```python
from build123d import *

# Parameters (mm, degrees)
SKETCH2_R               = 11.43
BOSS_EXTRUDE1_DEPTH     = 6.35
SKETCH4_R               = 1.5
CUT_EXTRUDE1_DEPTH      = 18.366988801
CUT_EXTRUDE2_REACH      = 29.445
CUT_EXTRUDE2_END_RADIUS = 1.5
CUT_EXTRUDE3_REACH      = 29.445
CUT_EXTRUDE3_END_RADIUS = 1.5
SKETCH9_R               = 1
SKETCH10_R              = 5.08
CUT_EXTRUDE4_DEPTH      = 3.81


with BuildPart() as part:
    # Sketch2 → Boss-Extrude1 (new body)
    with BuildSketch(Plane(origin=(0, 0, 0), x_dir=(1, 0, 0), z_dir=(0, 1, 0))):
        with Locations(Location((0, 0, 0), (0, 0, 270))):
            Circle(SKETCH2_R)
    extrude(amount=BOSS_EXTRUDE1_DEPTH)

    # Sketch4 → Cut-Extrude1 (cut, through all)
    with BuildSketch(Plane(origin=(0, 6.35, 0), x_dir=(1, 0, 0), z_dir=(0, 1, 0))):
        with Locations(Location((0, 8, 0), (0, 0, 270))):
            Circle(SKETCH4_R)
        with Locations(Location((0, -8, 0), (0, 0, 270))):
            Circle(SKETCH4_R)
        with Locations(Location((9.5, 0, 0), (0, 0, 270))):
            Circle(SKETCH4_R)
        with Locations(Location((-9.5, 0, 0), (0, 0, 270))):
            Circle(SKETCH4_R)
    extrude(amount=-CUT_EXTRUDE1_DEPTH, mode=Mode.SUBTRACT)

    # Cut-Extrude2: up to this cylinder (the profile starts outside it)
    cut_extrude2_end = Plane(origin=(0, 3.175, 8), z_dir=(0, 1, 0)) * Cylinder(CUT_EXTRUDE2_END_RADIUS, 62.89, mode=Mode.PRIVATE)
    # Sketch8 → Cut-Extrude2 (cut, up to the surface)
    with BuildSketch(Plane.XY.offset(12.7), mode=Mode.PRIVATE) as cut_extrude2_sk1:
        with BuildLine():
            ThreePointArc((1, 3.175), (0.707106781, 3.882106781), (0, 4.175))
            Line((0, 4.175), (0, 2.175))
            ThreePointArc((0, 2.175), (0.707106781, 2.467893219), (1, 3.175))
        make_face()
    cut_extrude2_tool1 = extrude(cut_extrude2_sk1.sketch, amount=-CUT_EXTRUDE2_REACH, mode=Mode.PRIVATE) - cut_extrude2_end
    add(cut_extrude2_tool1.solids().sort_by_distance((0.424413, 3.175, 12.7))[0], mode=Mode.SUBTRACT)
    # Sketch8 → Cut-Extrude2 (cut, up to the surface)
    with BuildSketch(Plane.XY.offset(12.7), mode=Mode.PRIVATE) as cut_extrude2_sk2:
        with BuildLine():
            Line((0, 2.175), (0, 4.175))
            ThreePointArc((0, 4.175), (-1, 3.175), (0, 2.175))
        make_face()
    cut_extrude2_tool2 = extrude(cut_extrude2_sk2.sketch, amount=-CUT_EXTRUDE2_REACH, mode=Mode.PRIVATE) - cut_extrude2_end
    add(cut_extrude2_tool2.solids().sort_by_distance((-0.424413, 3.175, 12.7))[0], mode=Mode.SUBTRACT)
    # Sketch8 → Cut-Extrude2 (cut, up to the surface)
    with BuildSketch(Plane.XY.offset(12.7), mode=Mode.PRIVATE) as cut_extrude2_sk3:
        with BuildLine():
            ThreePointArc((1, 3.175), (0.707106781, 3.882106781), (0, 4.175))
            Line((0, 4.175), (0, 2.175))
            ThreePointArc((0, 2.175), (0.707106781, 2.467893219), (1, 3.175))
        make_face()
    cut_extrude2_tool3 = extrude(cut_extrude2_sk3.sketch, amount=-CUT_EXTRUDE2_REACH, mode=Mode.PRIVATE) - cut_extrude2_end
    add(cut_extrude2_tool3.solids().sort_by_distance((0.424413, 3.175, 12.7))[0], mode=Mode.SUBTRACT)
    # Sketch8 → Cut-Extrude2 (cut, up to the surface)
    with BuildSketch(Plane.XY.offset(12.7), mode=Mode.PRIVATE) as cut_extrude2_sk4:
        with BuildLine():
            Line((0, 2.175), (0, 4.175))
            ThreePointArc((0, 4.175), (-1, 3.175), (0, 2.175))
        make_face()
    cut_extrude2_tool4 = extrude(cut_extrude2_sk4.sketch, amount=-CUT_EXTRUDE2_REACH, mode=Mode.PRIVATE) - cut_extrude2_end
    add(cut_extrude2_tool4.solids().sort_by_distance((-0.424413, 3.175, 12.7))[0], mode=Mode.SUBTRACT)

    # Cut-Extrude3: up to this cylinder (the profile starts outside it)
    cut_extrude3_end = Plane(origin=(0, 3.175, -8), z_dir=(0, 1, 0)) * Cylinder(CUT_EXTRUDE3_END_RADIUS, 62.89, mode=Mode.PRIVATE)
    # Sketch9 → Cut-Extrude3 (cut, up to the surface)
    with BuildSketch(Plane.XY.offset(-12.7), mode=Mode.PRIVATE) as cut_extrude3_sk1:
        with Locations(Location((0, 3.175, 0), (0, 0, 270))):
            Circle(SKETCH9_R)
    cut_extrude3_tool1 = extrude(cut_extrude3_sk1.sketch, amount=CUT_EXTRUDE3_REACH, mode=Mode.PRIVATE) - cut_extrude3_end
    add(cut_extrude3_tool1.solids().sort_by_distance((0, 3.175, -12.7))[0], mode=Mode.SUBTRACT)

    # Sketch10 → Cut-Extrude4 (cut)
    with BuildSketch(Plane(origin=(0, 6.35, 0), x_dir=(1, 0, 0), z_dir=(0, 1, 0))):
        with Locations(Location((0, 0, 0), (0, 0, 270))):
            Circle(SKETCH10_R)
    extrude(amount=-CUT_EXTRUDE4_DEPTH, mode=Mode.SUBTRACT)


solid = part.part
```
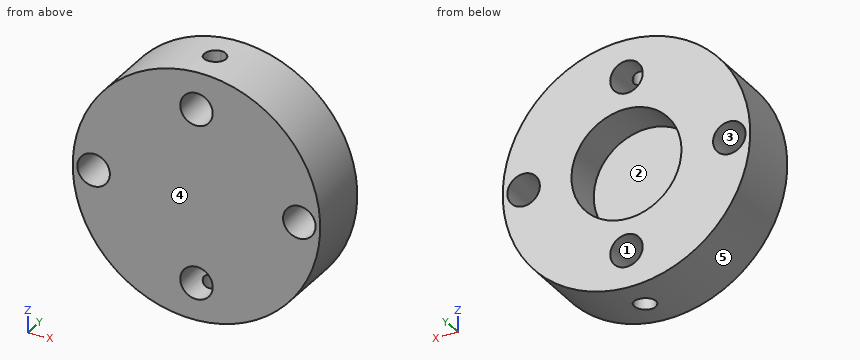
Work out the finished part from the listing and answer in its coordinate system (mm). Face numbers are marked on the shaded views. A direction names the side the tool comes from. Round coordinates to 2 decimals unless told otherwise and drop trailing zeros. Write each loop counter-clockwise with the first axis right and the second up, starting at its lowest first coordinate (ties: lowest second). Pieces come first, ordered by that corner, then holes. Notation, with made-up numbers: (80.5, 55) -> (99.5, 55) arc R10 cw to (99.5, 72) -> close; hole circle Ø6 at (-16.5, 9.5). An arc over 180 degrees is marked (long way). Write each question's results on one line, items separated by ' | '.
Q1. Section B-B, the plane z = 8 is taken. Write down the section's boundary in (x, y).
Data:
outline: (-8.16, 0) -> (-1.5, 0) -> (-1.5, 6.35) -> (-8.16, 6.35) -> close; (1.5, 0) -> (8.16, 0) -> (8.16, 6.35) -> (1.5, 6.35) -> close
Q2. Section D-D, the plane z = -0.75 is taken. Write down the section's boundary in (x, y).
Data:
outline: (-11.41, 0) -> (-10.8, 0) -> (-10.8, 6.35) -> (-11.41, 6.35) -> close; (-8.2, 0) -> (8.2, 0) -> (8.2, 6.35) -> (5.02, 6.35) -> (5.02, 2.54) -> (-5.02, 2.54) -> (-5.02, 6.35) -> (-8.2, 6.35) -> close; (10.8, 0) -> (11.41, 0) -> (11.41, 6.35) -> (10.8, 6.35) -> close
Q3. Flat-ended cylindrical pins translate along their axes: P1, Ø2, axis at x = -7.5, y = 3, coming from the +Z side; P2, Ø2, axis at x = 3, z = -1, coming from the +Y side; P3, Ø2.5, axis at x = 9.5, z = 0, coming from the -Y side; P4, Ø3, axis at x = -7.5, y = 3.5, coming from the -Z side. Find the tip coordinate at first contact, or state that the pin passes through.
Data:
P1: z = 9.4 | P2: y = 2.54 | P3: through | P4: z = -9.73
Q4. Determine the mould class of the marked faces 3, 4 and 5 for opening direction Z: released by +Z, released by -Z, zero draft, split by the parting line, or undercut.
Data:
face 3: undercut | face 4: zero draft | face 5: split by the parting line
Q5. Straight lines are drawn through the part: line 1 along X through (y, z) = (4, -0.5); line 2 along X through (y, z) = (3.75, -2.5); line 3 along X through (y, z) = (4, -8). For each, find the intervals that lie inside material, in ascending order. Write a range as [from, to].
Data:
line 1: [-11.42, -10.91], [-8.09, -5.06], [5.06, 8.09], [10.91, 11.42] | line 2: [-11.15, -4.42], [4.42, 11.15] | line 3: [-8.16, -1.5], [1.5, 8.16]
Q6. Section A-A, the plane x = -9 is taken. Write down the section's boundary in (y, z), then the cut area to 3 significant figures.
Data:
outline: (0, -7.05) -> (6.35, -7.05) -> (6.35, -1.41) -> (0, -1.41) -> close; (0, 1.41) -> (6.35, 1.41) -> (6.35, 7.05) -> (0, 7.05) -> close | area: 71.5 mm^2
Q7. Section C-C, the plane y = 1 is taken. Write down the section's boundary in (x, z), then the cut area to 3 significant figures.
Data:
outline: circle Ø22.86 at (0, 0); hole circle Ø3 at (-9.5, 0); hole circle Ø3 at (0, -8); hole circle Ø3 at (0, 8); hole circle Ø3 at (9.5, 0) | area: 382 mm^2
Q8. Which of the six approach directions +Z, -Z, +X, -X, +Y, -Y give full straight-line access (tool end or side, diameter ignored) to the marked faces 1 and 2?
Data:
face 1: +Y, -Y | face 2: +Y
